Verification items for the finished model (mm, model axes). Face numbers are marked on the shaded views. A direction names the side the tool comes from. Round coordinates to 2 decimals unless told otherwise and drop trailing zeros. Order: outer loops, then holes, each group sorted by start corner. A loop starts at its lowest first (then second) coordinate and runs counter-clockwise, first axis right, second up. Notation, with made-up numbers: (55, 19.5) -> (102, 19.5) arc R16 cw to (102, 24.5) -> close; hole circle Ø11 at (19, 84). An arc over 180 degrees is marked (long way). Return JSON: item names as keys, results as strings. Group by question number.
Item 1: Depth check by flat-ended pin: pin 1 Ø1.2 at (y, z) = (1.5, -7.5) entering from +X. Enter the tip coordinate at first touch or a pass-through.
Item 2: Sectioned sample at B-B on x = 10.5. Record the cut outline in (y, z), plus the area to 3 significant figures.
Item 3: Scan lines: probe 1 along Z at (x, y) = (11.75, 0.35); probe 2 along X at (y, z) = (2.7, -11.5); probe 3 along Z at (x, y) = (0.5, 2.4). Record each from-to range of solid material in increasing order. Write a range as from..to.
Item 4: Access from +Z, -Z, +X, -X, +Y, -Y to the whole of each face (thin tool, end or side, straight path). Record for the marked faces 1 and 2.
Item 5: Sectioned sample at A-A on y = 0.7. Record the cut outline in (x, z), plus the area to 3 significant figures.
Item 6: Sectioned sample at C-C on z = -8.25. Record the cut outline in (x, y).
```python
from build123d import *

# Parameters (mm, degrees)
BOSS_EXTRUDE1_DEPTH = 4
FILLET1_R           = 1


with BuildPart() as part:
    # Sketch1 → Boss-Extrude1 (new body)
    with BuildSketch(Plane(origin=(0, 0, 0), x_dir=(1, 0, 0), z_dir=(0, 1, 0))):
        Polygon((0, 0), (12, 0), (12, 2), (2, 2), (2, 12), (0, 12), align=None)
    extrude(amount=BOSS_EXTRUDE1_DEPTH)

    # Fillet1
    fillet1_edges = [part.edges().sort_by_distance(p)[0] for p in [
        (0, 2, 0),
    ]]
    fillet(fillet1_edges, radius=FILLET1_R)


solid = part.part
```
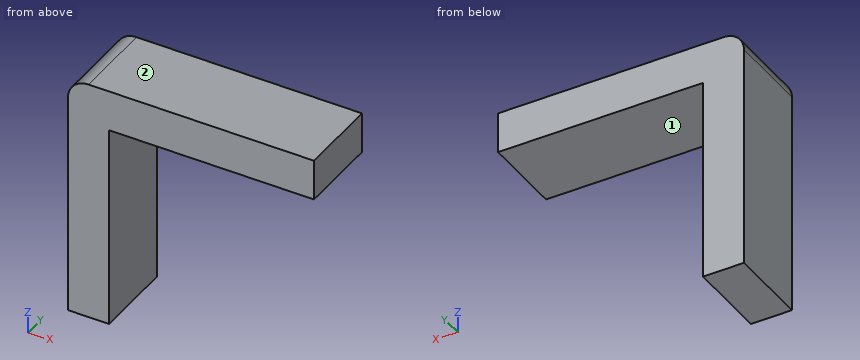
Recorded:
{
 "1": {"pin 1": "x = 2"},
 "2": {"outline": "(0, -2) -> (4, -2) -> (4, 0) -> (0, 0) -> close", "area": "8.00 mm²"},
 "3": {"probe 1": "-2..0", "probe 2": "0..2", "probe 3": "-12..-0.13"},
 "4": {"face 1": "-Z, +X, +Y, -Y", "face 2": "+Z, +X, -X, +Y, -Y"},
 "5": {"outline": "(0, -12) -> (2, -12) -> (2, -2) -> (12, -2) -> (12, 0) -> (1, 0) arc R1 ccw to (0, -1) -> close", "area": "43.8 mm²"},
 "6": {"outline": "(0, 0) -> (2, 0) -> (2, 4) -> (0, 4) -> close"}
}
